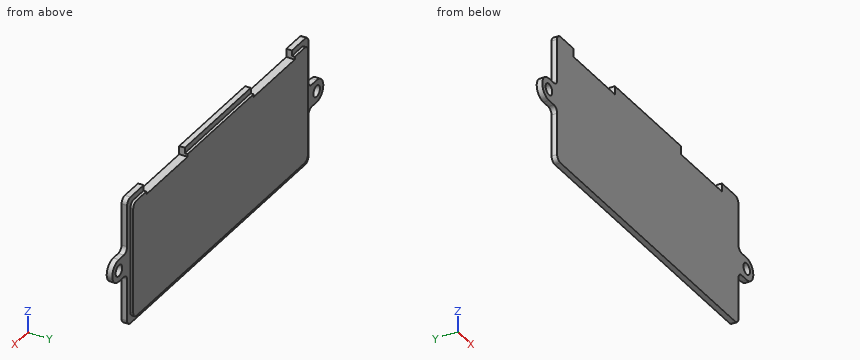
Autodesk Inventor part; units mm, degrees
ref_plane "Work Plane1" through (64, 2, 0) normal (0, 0, -1) x (-1, 0, 0)
ref_plane "Work Plane2" through (0, 2, -23) normal (-1, 0, 0) x (0, -1, 0)
ref_plane "YZ Plane" through (0, 0, 0) normal (1, 0, 0) x (0, 1, 0)
sketch "Sketch1" plane through (0, 0, 0) normal (0, 1, 0) x (-1, 0, 0)
  line L0 (55, 23) -> (-55, 23)
  line L1 (-55, 23) -> (-55, -23)
  line L2 (-55, -23) -> (55, -23)
  line L3 (55, -23) -> (55, 23)
  line L4 (55, 23) -> (-55, -23) construction
  line L5 (-55, 23) -> (55, -23) construction
  circle A0 centre (60, 0) radius 2
  circle A1 centre (-60, 0) radius 2
  arc A2 (60, -4) -> (60, 4) centre (60, 0) ccw
  line L6 (55, -4) -> (60, -4)
  line L7 (60, 4) -> (55, 4)
  line L8 (55, 4) -> (55, -4)
  arc A3 (-60, 4) -> (-60, -4) centre (-60, 0) ccw
  line L9 (-55, -4) -> (-60, -4)
  line L10 (-60, 4) -> (-55, 4)
  line L11 (-55, 4) -> (-55, -4)
  point P0 (0, 0)
  point P1 (55, 0)
  point P2 (-55, 0)
  point P3 (55, 0)
  point P4 (-55, 0)
  dimension "d0" = 110
  dimension "d1" = 46
  dimension "d2" = 4
  dimension "d3" = 5
  dimension "d4" = 4
  dimension "d5" = 5
  dimension "d6" = 8
  dimension "d7" = 5
  dimension "d8" = 4
  dimension "d9" = 8
  dimension "d10" = 5
  dimension "d11" = 4
extrude "Extrusion1" add sketch "Sketch1" along normal blind 2
sketch "Sketch2" plane through (0, 2, 0) normal (0, 1, 0) x (1, 0, 0)
  line L0 (-53, -21) -> (53, -21)
  line L1 (53, -21) -> (53, 21)
  line L2 (53, 21) -> (-53, 21)
  line L3 (-53, 21) -> (-53, -21)
  line L4 (-53, -21) -> (53, 21) construction
  line L5 (53, -21) -> (-53, 21) construction
  point P0 (0, 0)
  dimension "d14" = 106
  dimension "d15" = 42
extrude "Extrusion2" add sketch "Sketch2" along normal blind 1
fillet "Fillet1" radius 2 12 edges at (53, 2.5, 21) (55, 1, 23) (55, 1, 4) (55, 1, -4) (55, 1, -23) (53, 2.5, -21) (-55, 1, -23) (-53, 2.5, -21) (-55, 1, -4) (-55, 1, 4) (-53, 2.5, 21) (-55, 1, 23)
sketch "Sketch3" plane through (0, 0, 0) normal (0, -1, 0) x (1, 0, 0)
  line L0 (-53, 23) -> (53, 23)
  line L1 (-45, 23) -> (-20, 23)
  line L2 (-20, 23) -> (-20, 20)
  line L3 (-20, 20) -> (-45, 20)
  line L4 (-45, 20) -> (-45, 23)
  line L5 (20, 23) -> (45, 23)
  line L6 (45, 23) -> (45, 20)
  line L7 (45, 20) -> (20, 20)
  line L8 (20, 20) -> (20, 23)
  line L9 (-55, 6) -> (-55, 21)
  line L10 (55, 21) -> (55, 6)
  point P0 (0, 0)
  point P1 (-45, 21.5)
  point P2 (45, 21.5)
  dimension "d19" = 25
  dimension "d20" = 3
  dimension "d21" = 25
  dimension "d22" = 3
  dimension "d23" = 10
  dimension "d24" = 10
extrude "Extrusion3" cut sketch "Sketch3" against normal through all
ref_plane "Work Plane1" through (64, 2, 0) normal (0, 0, -1) x (-1, 0, 0)
ref_plane "Work Plane2" through (0, 2, -23) normal (-1, 0, 0) x (0, -1, 0)
properties part number "StereoPiBracketLid"
For this review, take the finished solid that the model builds, in its own axes (mm). Give positions to 0.01 mm unless a question says otherwise; leave off trailing zeros. Loops run counter-clockwise (first coordinate to the right, second up) from the corner with the lowest first, then second, coordinate; pieces in that order, holes last.
Item 1: Take a section at C-C, the plane x = 13. State the section outline as (y, z) points, and give its area (3 significant figures).
Item 2: Take a section at B-B, the plane z = -13. State the section outline as (x, y) points.
Item 3: Take a section at A-A, the plane y = 1.1. Give the number of separate pieces and of enclosed holes in the cut face, and give its area (3 significant figures).
Item 4: Insertion check: pin 1 (0.6 mm diameter, centred on y = 1, z = 17, fed in from -X); pin 2 (1.5 mm diameter, centred on y = 2, z = 21, fed in from +X); pin 3 (0.8 mm diameter, centred on x = 47, y = 2.5, fed in from +Z). Each pin has a flat end and moves straight along its axis. Give the tip position at first contact, or say it passes through.
Item 5: For line 1 along Z through (x, y) = (60, 1.5); line 2 along X through (y, z) = (0.2, -1); line 3 along X through (y, z) = (2.9, 13), list the stretches that pass through material, from the lowest coordinate up.
Calculated:
1. outline: (0, -23) - (2, -23) - (2, -21) - (3, -21) - (3, 21) - (2, 21) - (2, 23) - (0, 23) - close
1. area: 134 mm2
2. outline: (-55, 0) - (55, 0) - (55, 2) - (53, 2) - (53, 3) - (-53, 3) - (-53, 2) - (-55, 2) - close
3. separate pieces: 1
3. enclosed holes: 2
3. area: 5,020 mm2
4. pin 1: stops at x = -55
4. pin 2: stops at x = 55
4. pin 3: stops at z = 21
5. line 1: z = -4 to -2, 2 to 4
5. line 2: x = -63.87 to -61.73, -58.27 to 58.27, 61.73 to 63.87
5. line 3: x = -53 to 53
